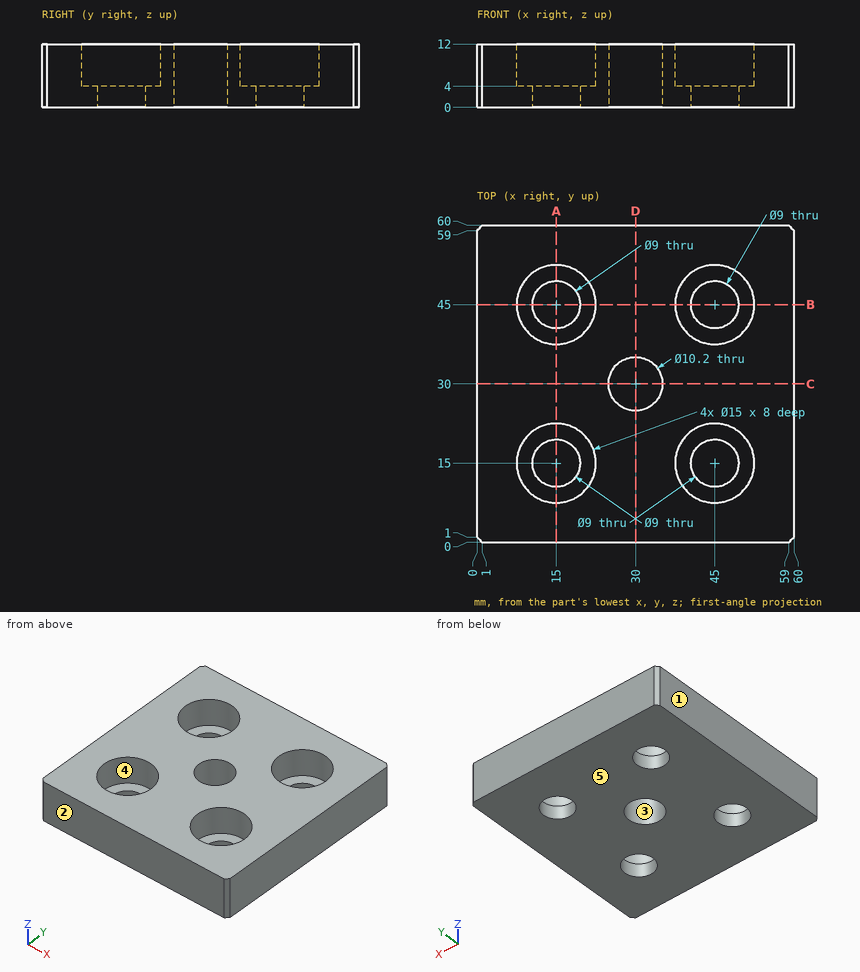
Print and shaded views of the part. All mm, measured from the part's lowest x, y and z. A direction names the side the tool comes from. Give positions to 0.01 mm unless a question says otherwise; leave off trailing zeros. Order: outer loops, then holes, each group sorted by start corner. A loop starts at its lowest first (then second) coordinate and runs counter-clockwise, first axis right, second up. Notation, with made-up numbers: M 75,3.25 L 102,3.25 A26 cw 102,20.25 Z; hole C 41,-29.75 d7. An arc over 180 degrees is marked long. Use one line per item in the form item = value.
Q1. Wall check: probe 1 along X at (y, z) = (44.5, 9.75); probe 2 along Y at (x, z) = (45, 3.2); probe 3 along Y at (x, z) = (45, 9). Give the ranges that are in metal, low to high.
Conclusion:
probe_1 = 0 to 7.52, 22.48 to 37.52, 52.48 to 60
probe_2 = 0 to 10.5, 19.5 to 40.5, 49.5 to 60
probe_3 = 0 to 7.5, 22.5 to 37.5, 52.5 to 60
Q2. Which spindle directions (+Z, -Z, +X, -X, +Y, -Y) get a long thin tool onto all of the face, cutting with end or side? Do the marked faces 4 and 5. Say none if no direction does.
Conclusion:
face_4 = +Z
face_5 = -Z, +X, -X, +Y, -Y
Q3. Slice it at A-A, the plane x = 15. Write the cut outline in (y, z), and give its area (3 significant figures).
Conclusion:
outline = M 0,0 L 10.5,0 L 10.5,4 L 7.5,4 L 7.5,12 L 0,12 Z; M 19.5,0 L 40.5,0 L 40.5,4 L 37.5,4 L 37.5,12 L 22.5,12 L 22.5,4 L 19.5,4 Z; M 49.5,0 L 60,0 L 60,12 L 52.5,12 L 52.5,4 L 49.5,4 Z
area = 408 mm2
Q4. Slice it at C-C, the plane y = 30. Write the cut outline in (x, z).
Conclusion:
outline = M 0,0 L 24.9,0 L 24.9,12 L 0,12 Z; M 35.1,0 L 60,0 L 60,12 L 35.1,12 Z
Q5. Pin check, flat tip, straight feed: P1, Ø7.5, axis at x = 17.5, y = 47, coming from the +Z side. Stop position of the tip, or through.
Conclusion:
P1 = 4
Q6. Pull direction Y, two halves, no side cores. Call the marked faces 1, 2 and 3: released by +Y, released by -Y, zero draft, split by the parting line, or undercut.
Conclusion:
face_1 = zero draft
face_2 = released by -Y
face_3 = undercut
